The listing builds one solid part. Answer for the finished solid, in the listing's coordinates (mm). Give positions to 0.01 mm unless a question says otherwise; leave off trailing zeros. Loops run counter-clockwise (first coordinate to the right, second up) from the corner with the lowest first, then second, coordinate; pieces in that order, holes last. Notation, with made-up numbers: M 21,80.5 L 41,80.5 A26 cw 41,113.5 Z; hole C -23.5,-35 d3. An arc over 180 degrees is marked long. Use one line per item in the form item = value. Start each with the question number.
1. The part is cut by section B-B (x = 17.5). Write down the section's boundary in (y, z), and give its area (3 significant figures).
2. Each of these flat-tipped pins is pushed along its axis until it touches: pin 1 Ø4 at (x, z) = (-17.5, -12.5) entering from +Y; pin 2 Ø0.6 at (x, y) = (0, 4.5) entering from +Z. Where does it stop, or does it pass through?
3. The part is cut by section D-D (x = -7). Write down the section's boundary in (y, z).
4. Straight lines are drawn through the part: line 1 (Z direction, x = -17.5, y = 0.85); line 2 (X direction, y = 1.85, z = 12.5); line 3 (Z direction, x = 18.5, y = 1.75). For each, find the intervals that lie inside material, in ascending order. Write a range as from..to.
5. The part is cut by section A-A (z = -12.5). Write down the section's boundary in (x, y).
6. The part is cut by section C-C (y = 2). Write down the section's boundary in (x, z), and give its area (3 significant figures).
from build123d import *

# Parameters (mm, degrees)
SKETCH1_W     = 50
SKETCH1_H     = 40
BODY_DEPTH    = 3
FILLET_BODY_R = 3
SKETCH2_R     = 1.5
BOLTS_DEPTH   = 9
SKETCH3_W     = 15.5
SKETCH3_H     = 9.5
CHANNEL_DEPTH = 2


with BuildPart() as part:
    # Sketch1 → Body (new body)
    with BuildSketch(Plane(origin=(0, 0, 0), x_dir=(1, 0, 0), z_dir=(0, 1, 0))):
        Rectangle(SKETCH1_W, SKETCH1_H)
    extrude(amount=BODY_DEPTH)

    # Fillet_Body
    fillet_body_edges = [part.edges().sort_by_distance(p)[0] for p in [
        (-25, 1.5, -20),
        (25, 1.5, -20),
        (25, 1.5, 20),
        (-25, 1.5, 20),
    ]]
    fillet(fillet_body_edges, radius=FILLET_BODY_R)

    # Sketch2 → Bolts (cut)
    with BuildSketch(Plane(origin=(0, 3, 0), x_dir=(1, 0, 0), z_dir=(0, 1, 0))):
        with Locations((-17.5, 12.5)):
            Circle(SKETCH2_R)
        with Locations((17.5, 12.5)):
            Circle(SKETCH2_R)
        with Locations((17.5, -12.5)):
            Circle(SKETCH2_R)
        with Locations((-17.5, -12.5)):
            Circle(SKETCH2_R)
    extrude(amount=-BOLTS_DEPTH, mode=Mode.SUBTRACT)

    # Sketch3 → Channel (add)
    with BuildSketch(Plane(origin=(0, 3, 0), x_dir=(1, 0, 0), z_dir=(0, 1, 0))):
        Rectangle(SKETCH3_W, SKETCH3_H)
    extrude(amount=CHANNEL_DEPTH)


solid = part.part
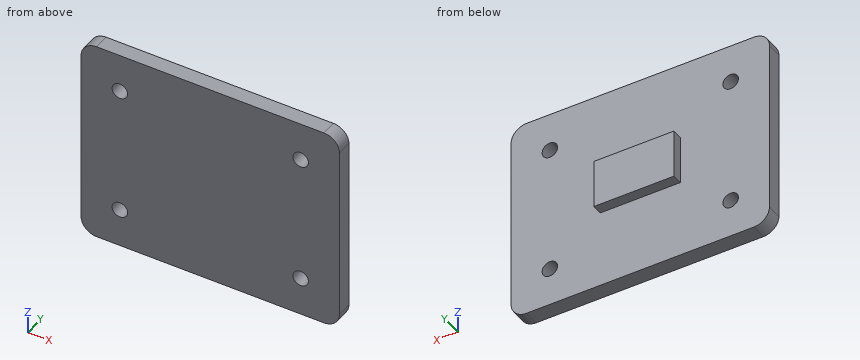
Derived:
q1.outline = M 0,-20 L 3,-20 L 3,-14 L 0,-14 Z; M 0,-11 L 3,-11 L 3,11 L 0,11 Z; M 0,14 L 3,14 L 3,20 L 0,20 Z
q1.area = 102 mm2
q2.pin_1 = 3
q2.pin_2 = 4.75
q3.outline = M 0,-20 L 3,-20 L 3,-4.75 L 5,-4.75 L 5,4.75 L 3,4.75 L 3,20 L 0,20 Z
q4.line_1 = -20..-14, -11..11, 14..20
q4.line_2 = -25..-19, -16..16, 19..25
q4.line_3 = -20..-13.62, -11.38..11.38, 13.62..20
q5.outline = M -25,0 L -19,0 L -19,3 L -25,3 Z; M -16,0 L 16,0 L 16,3 L -16,3 Z; M 19,0 L 25,0 L 25,3 L 19,3 Z
q6.outline = M -25,-17 A3 ccw -22,-20 L 22,-20 A3 ccw 25,-17 L 25,17 A3 ccw 22,20 L -22,20 A3 ccw -25,17 Z; hole C -17.5,-12.5 d3; hole C -17.5,12.5 d3; hole C 17.5,-12.5 d3; hole C 17.5,12.5 d3
q6.area = 1,960 mm2
